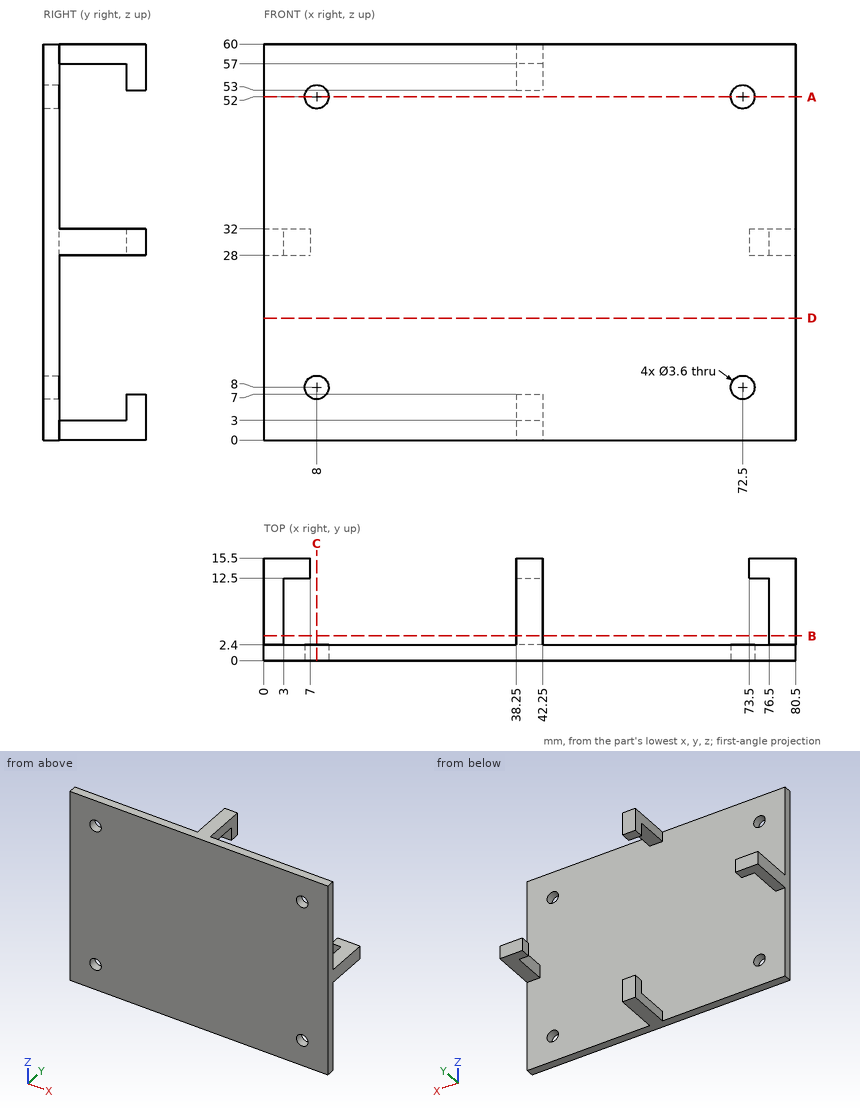
Here's the drawing with two shaded views (mm, measured from the low corner). I have some questions. Give positions to 0.01 mm unless a question says otherwise; leave off trailing zeros. Order: outer loops, then holes, each group sorted by start corner. A loop starts at its lowest first (then second) coordinate and runs counter-clockwise, first axis right, second up. Notation, with made-up numbers: (35.5, -28.5) - (47.5, -28.5) arc R26 cw to (47.5, 2.5) - close; hole circle Ø10 at (-36, 69.5). An arc over 180 degrees is marked (long way). Write each question's results on one line, items separated by ' | '.
1) Please list where these lines run through material, in increasing order: line 1 along Z through (x, y) = (72.5, 1.8); line 2 along X through (y, z) = (1.35, 8); line 3 along X through (y, z) = (5.5, 29.5). Write a range as [from, to].
Final values:
line 1: z = [0, 6.2], [9.8, 50.2], [53.8, 60] | line 2: x = [0, 6.2], [9.8, 70.7], [74.3, 80.5] | line 3: x = [0, 3], [76.5, 80.5]
2) Suppose I cut it at B-B, the plane y = 3.75. Write out the boundary of the cut face in (x, z).
Final values:
outline: (0, 28) - (3, 28) - (3, 32) - (0, 32) - close; (38.25, 0) - (42.25, 0) - (42.25, 3) - (38.25, 3) - close; (38.25, 57) - (42.25, 57) - (42.25, 60) - (38.25, 60) - close; (76.5, 28) - (80.5, 28) - (80.5, 32) - (76.5, 32) - close
3) Suppose I cut it at A-A, the plane z = 52. Write out the boundary of the cut face in (x, y).
Final values:
outline: (0, 0) - (6.2, 0) - (6.2, 2.4) - (0, 2.4) - close; (9.8, 0) - (70.7, 0) - (70.7, 2.4) - (9.8, 2.4) - close; (74.3, 0) - (80.5, 0) - (80.5, 2.4) - (74.3, 2.4) - close
4) Suppose I cut it at D-D, the plane z = 18.5. Write out the boundary of the cut face in (x, y), then the cut area to 3 significant figures.
Final values:
outline: (0, 0) - (80.5, 0) - (80.5, 2.4) - (0, 2.4) - close | area: 193 mm^2
5) I'm going to push flat-ended pins straight in: pin 1 Ø5.5 at (x, y) = (78, 6.5) entering from -Z; pin 2 Ø1.5 at (x, z) = (41, 11) entering from +Y; pin 3 Ø4.5 at (x, z) = (8, 52) entering from -Y; pin 4 Ø2 at (y, z) = (10, 57) entering from -X. Where does each tip first touch, or does it pass through?
Final values:
pin 1: stops at z = 28 | pin 2: stops at y = 2.4 | pin 3: stops at y = 0 | pin 4: stops at x = 38.25
6) Suppose I cut it at C-C, the plane x = 8. Write out the boundary of the cut face in (y, z), then the cut area to 3 significant figures.
Final values:
outline: (0, 0) - (2.4, 0) - (2.4, 6.2) - (0, 6.2) - close; (0, 9.8) - (2.4, 9.8) - (2.4, 50.2) - (0, 50.2) - close; (0, 53.8) - (2.4, 53.8) - (2.4, 60) - (0, 60) - close | area: 127 mm^2
